```python
from build123d import *

# Parameters (mm, degrees)
F1_DEPTH = 3.4
F2_DEPTH = 10
F3_R     = 2


with BuildPart() as f1:
    # F0 (on Top) → F1 (new body)
    with BuildSketch(Plane.XY):
        with BuildLine():
            ThreePointArc((18.943376, 38.95781), (17.113249, 40.787937), (14.613249, 41.45781))
            Line((14.613249, 41.45781), (-14.613249, 41.45781))
            ThreePointArc((-14.613249, 41.45781), (-17.113249, 40.787937), (-18.943376, 38.95781))
            Line((-18.943376, 38.95781), (-43.210141, -3.07346))
            ThreePointArc((-43.210141, -3.07346), (-43.880014, -5.57346), (-43.210141, -8.07346))
            Line((-43.210141, -8.07346), (-28.596892, -33.38435))
            ThreePointArc((-28.596892, -33.38435), (-26.766765, -35.214477), (-24.266765, -35.88435))
            Line((-24.266765, -35.88435), (24.266765, -35.88435))
            ThreePointArc((24.266765, -35.88435), (26.766765, -35.214477), (28.596892, -33.38435))
            Line((28.596892, -33.38435), (43.210141, -8.07346))
            ThreePointArc((43.210141, -8.07346), (43.880014, -5.57346), (43.210141, -3.07346))
            Line((43.210141, -3.07346), (18.943376, 38.95781))
        make_face()
    extrude(amount=F1_DEPTH)

    # F0 (on Top) → F2 (join)
    with BuildSketch(Plane.XY):
        with BuildLine():
            Line((44.942192, -2.07346), (20.675426, 39.95781))
            ThreePointArc((20.675426, 39.95781), (18.113249, 42.519988), (14.613249, 43.45781))
            Line((14.613249, 43.45781), (-14.613249, 43.45781))
            ThreePointArc((-14.613249, 43.45781), (-18.113249, 42.519988), (-20.675426, 39.95781))
            Line((-20.675426, 39.95781), (-44.942192, -2.07346))
            ThreePointArc((-44.942192, -2.07346), (-45.880014, -5.57346), (-44.942192, -9.07346))
            Line((-44.942192, -9.07346), (-30.328943, -34.38435))
            ThreePointArc((-30.328943, -34.38435), (-27.766765, -36.946527), (-24.266765, -37.88435))
            Line((-24.266765, -37.88435), (24.266765, -37.88435))
            ThreePointArc((24.266765, -37.88435), (27.766765, -36.946527), (30.328943, -34.38435))
            Line((30.328943, -34.38435), (44.942192, -9.07346))
            ThreePointArc((44.942192, -9.07346), (45.880014, -5.57346), (44.942192, -2.07346))
        make_face()
        with BuildLine():
            Line((-14.613249, 41.45781), (14.613249, 41.45781))
            ThreePointArc((14.613249, 41.45781), (17.113249, 40.787937), (18.943376, 38.95781))
            Line((18.943376, 38.95781), (43.210141, -3.07346))
            ThreePointArc((43.210141, -3.07346), (43.880014, -5.57346), (43.210141, -8.07346))
            Line((43.210141, -8.07346), (28.596892, -33.38435))
            ThreePointArc((28.596892, -33.38435), (26.766765, -35.214477), (24.266765, -35.88435))
            Line((24.266765, -35.88435), (-24.266765, -35.88435))
            ThreePointArc((-24.266765, -35.88435), (-26.766765, -35.214477), (-28.596892, -33.38435))
            Line((-28.596892, -33.38435), (-43.210141, -8.07346))
            ThreePointArc((-43.210141, -8.07346), (-43.880014, -5.57346), (-43.210141, -3.07346))
            Line((-43.210141, -3.07346), (-18.943376, 38.95781))
            ThreePointArc((-18.943376, 38.95781), (-17.113249, 40.787937), (-14.613249, 41.45781))
        make_face(mode=Mode.SUBTRACT)
    extrude(amount=F2_DEPTH)

    # F3
    f3_edges = [f1.edges().sort_by_distance(p)[0] for p in [
        (32.808809, 18.942175, 0),
    ]]
    fillet(f3_edges, radius=F3_R)


solid = f1.part
```
The model under review builds one solid part; all positions refer to its coordinate system, in mm. A direction names the side the tool comes from. Coordinates: 2 decimals unless noted, no trailing zeros. Loops run counter-clockwise (first coordinate to the right, second up) from the corner with the lowest first, then second, coordinate; pieces in that order, holes last. Notation, with made-up numbers: (49.25, 39.25) -> (95.25, 39.25) arc R22 cw to (95.25, 55.25) -> close; hole circle Ø9 at (33.25, 57). An arc over 180 degrees is marked (long way). Answer as CSV lines item,"result".
Item 1: Draft analysis for pull direction X (two halves, no side actions). For faces 3 (the cylindrical face through (-18.069, 42.545, 5.944)), 4 (the cylindrical face through (32.145, 18.951, 0.601)), 5 (the flat face through (0, 41.458, 7)), state which applies: +X half, -X half, draft (parallel to the pull), parting line (faces both ways), or undercut.
Results below:
face 3,"-X half"
face 4,"+X half"
face 5,"undercut"
Item 2: Insertion check: pin 1 (6 mm diameter, centred on x = 27, y = -5, fed in from +Z); pin 2 (3 mm diameter, centred on y = -1, z = 7, fed in from -X); pin 3 (6 mm diameter, centred on y = -0.5, z = 7, fed in from +X). Each pin has a flat end and moves straight along its axis. Give the tip position at first contact, or say it passes through.
Results below:
pin 1,"stops at z = 3.4"
pin 2,"stops at x = -45.17"
pin 3,"stops at x = 45.57"
Item 3: Take a section at A-A, the plane z = 5.75. State the section outline as (x, y) points.
Results below:
outline,"(-44.94, -9.07) -> (-30.33, -34.38) arc R7 ccw to (-24.27, -37.88) -> (24.27, -37.88) arc R7 ccw to (30.33, -34.38) -> (44.94, -9.07) arc R7 ccw to (44.94, -2.07) -> (20.68, 39.96) arc R7 ccw to (14.61, 43.46) -> (-14.61, 43.46) arc R7 ccw to (-20.68, 39.96) -> (-44.94, -2.07) arc R7 ccw to start; hole (-43.21, -8.07) -> (-28.6, -33.38) arc R5 ccw to (-24.27, -35.88) -> (24.27, -35.88) arc R5 ccw to (28.6, -33.38) -> (43.21, -8.07) arc R5 ccw to (43.21, -3.07) -> (18.94, 38.96) arc R5 ccw to (14.61, 41.46) -> (-14.61, 41.46) arc R5 ccw to (-18.94, 38.96) -> (-43.21, -3.07) arc R5 ccw to start"
Item 4: Machinability: for faces 1 (the flat face through (-31.247, 17.648, 6.654)), 2 (the cylindrical face through (-45.88, -5.52, 5.94)), which of the approach directions +Z, -Z, +X, -X, +Y, -Y give a long, thin tool a straight path to every point of the face, cutting with its end or side? Answer none if there is none.
Results below:
face 1,"+Z"
face 2,"+Z, -Z, -X"
Item 5: For L1, parallel to Y at x = 8.5, z = 4.5; L2, parallel to Z at x = -10.5, y = -33.5; L3, parallel to Y at x = -28, z = 6.25, list the stretches that pass through material, from the lowest coordinate up.
Results below:
L1,"y = -37.88 to -35.88, 41.46 to 43.46"
L2,"z = 0 to 3.4"
L3,"y = -36.81 to -34.21, 23.27 to 27.27"
